Part model, mm, in its own coordinate system. Round coordinates to 2 decimals unless told otherwise and drop trailing zeros. Write each loop counter-clockwise with the first axis right and the second up, starting at its lowest first coordinate (ties: lowest second). Pieces come first, ordered by that corner, then holes. Notation, with made-up numbers: (-11.75, -13) -> (-4.75, -13) arc R5 ccw to (-4.75, -9) -> close; hole circle Ø4 at (-22.75, 31). An arc over 180 degrees is marked (long way). Use CSV: the item, a comma, the result in double quotes. Start each with the question number.
(1) Saw through at C-C (y = 4). Give the cut face in (x, z), plus the area to 3 significant figures.
(2) Probe line 1 (Y direction, x = 3.75, z = 0.2); line 2 (Y direction, x = 0, z = 0.3); line 3 (X direction, y = -4.75, z = 0.55). List the from-to ranges inside material, lowest first. Write a range as [from, to].
(3) Two-plate mould, pull along Y, no slides. Class faces 1 (the cylindrical face through (3.45, 3.63, 0.51)), 2 (the cylindrical face through (0, -6, 0.5)), 3 (the cylindrical face through (0.338, 8.994, 0.507)): released by +Y, released by -Y, zero draft, split by the parting line, or undercut.
(4) Saw through at B-B (x = 0). Give the cut face in (y, z), plus the area to 3 significant figures.
(5) Drop a flat-ended pin along its axis: pin 1 (1.6 mm diameter, centred on x = -4.24, y = 4.24, fed in from -Z) (1 decimal). Give the stop position or say it passes through.
(6) Saw through at D-D (z = 0.6). Count the separate pieces of the cut face and the enclosed holes in it, plus the area to 3 significant figures.
(7) Saw through at A-A (y = 0). Give the cut face in (x, z), plus the area to 3 significant figures.
```python
from build123d import *

# Parameters (mm, degrees)
F0_R     = 9
F0_R_2   = 1
F0_R_3   = 2.5
F2_R     = 3
F4_DEPTH = 1.001
F5_R     = 1


with BuildPart() as f3:
    # F3: sweep along a path in F1
    with BuildLine(Plane.XZ) as f3_path:
        Line((0, 0), (0, 1))
    # F0 (on Top) → F3 (sweep)
    with BuildSketch(Plane.XY):
        Circle(F0_R)
        with Locations((-4.2426406871, -4.2426406871)):
            Circle(F0_R_2, mode=Mode.SUBTRACT)
        with Locations((4.2426406871, -4.2426406871)):
            Circle(F0_R_2, mode=Mode.SUBTRACT)
        with Locations((-4.2426406871, 4.2426406871)):
            Circle(F0_R_2, mode=Mode.SUBTRACT)
        Circle(F0_R_3, mode=Mode.SUBTRACT)
        with Locations((4.2426406871, 4.2426406871)):
            Circle(F0_R_2, mode=Mode.SUBTRACT)
    sweep(path=f3_path.line)

    # F2 (on Top) → F4 (cut, through all)
    with BuildSketch(Plane.XY):
        with Locations((0, -9)):
            Circle(F2_R)
    extrude(amount=F4_DEPTH, mode=Mode.SUBTRACT)

    # F5
    f5_edges = [f3.edges().sort_by_distance(p)[0] for p in [
        (-2.95804, -8.5, 0.5),
        (2.95804, -8.5, 0.5),
    ]]
    fillet(f5_edges, radius=F5_R)


solid = f3.part
```
Answers:
1,outline,"(-8.06, 0) -> (-5.21, 0) -> (-5.21, 1) -> (-8.06, 1) -> close; (-3.27, 0) -> (3.27, 0) -> (3.27, 1) -> (-3.27, 1) -> close; (5.21, 0) -> (8.06, 0) -> (8.06, 1) -> (5.21, 1) -> close"
1,area,"12.2 mm²"
2,line 1,"y = [-8.15, -5.11], [-3.37, 3.37], [5.11, 8.18]"
2,line 2,"y = [-6, -2.5], [2.5, 9]"
2,line 3,"x = [-7.64, -5.1], [-3.38, 3.38], [5.1, 7.64]"
3,face 1,"undercut"
3,face 2,"released by -Y"
3,face 3,"split by the parting line"
4,outline,"(-6, 0) -> (-2.5, 0) -> (-2.5, 1) -> (-6, 1) -> close; (2.5, 0) -> (9, 0) -> (9, 1) -> (2.5, 1) -> close"
4,area,"10.0 mm²"
5,pin 1,"passes through"
6,separate pieces,"1"
6,enclosed holes,"5"
6,area,"209 mm²"
7,outline,"(-9, 0) -> (-2.5, 0) -> (-2.5, 1) -> (-9, 1) -> close; (2.5, 0) -> (9, 0) -> (9, 1) -> (2.5, 1) -> close"
7,area,"13.0 mm²"
